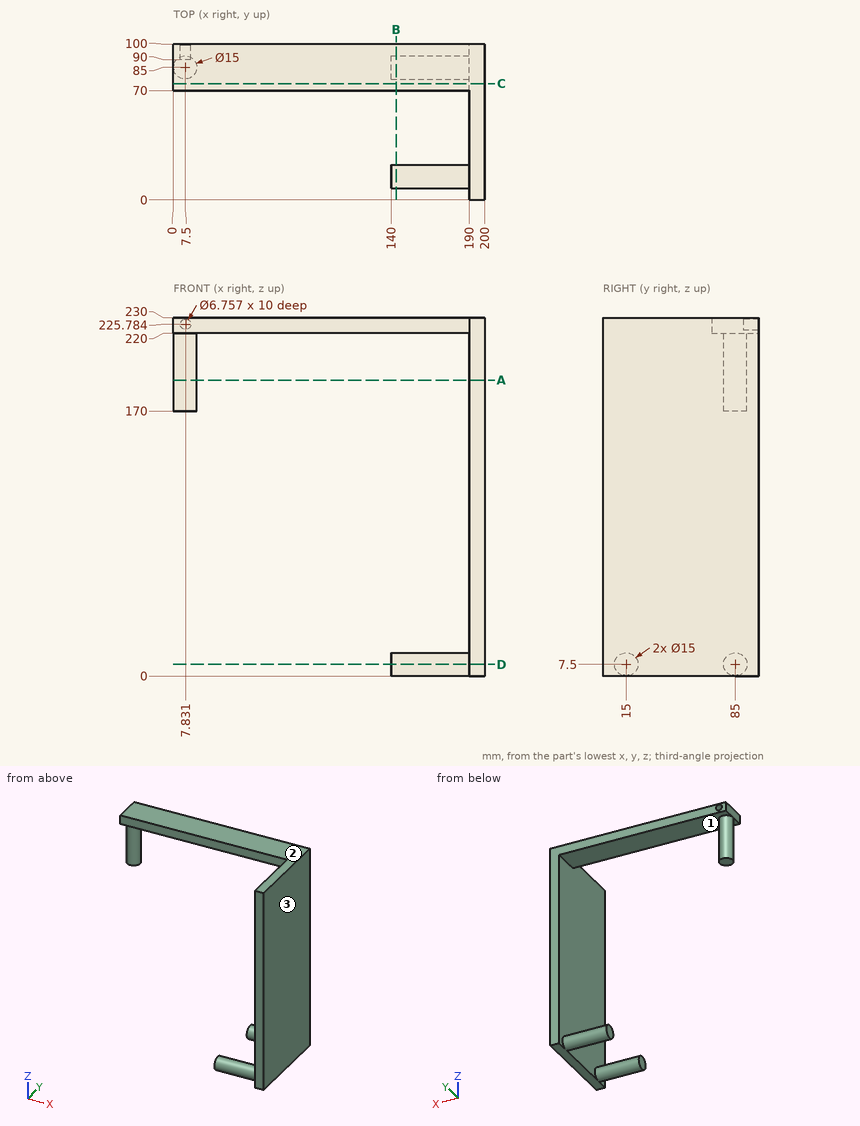
The drawing under review shows one solid part. Ordinate dimensions are in mm from its lowest x, y, z. Give positions to 0.01 mm unless a question says otherwise; leave off trailing zeros. Write each loop counter-clockwise with the first axis right and the second up, starting at its lowest first coordinate (ties: lowest second). Pieces come first, ordered by that corner, then holes. Notation, with made-up numbers: M 66.5,87 L 72.5,87 A10 ccw 72.5,92 Z; hole C 79,-6.5 d3. An arc over 180 degrees is marked long. Write each question's results on one line, items separated by ' | '. Start each with the question number.
1. We need section A-A (z = 190). Write out the cut boundary in (x, y), and give its area (3 significant figures).
2. We need section D-D (z = 7.5). Write out the cut boundary in (x, y).
3. Insertion check: pin 1 Ø7.5 at (y, z) = (84.5, 8.5) entering from -X; pin 2 Ø7.5 at (x, y) = (6, 88) entering from -Z; pin 3 Ø5.5 at (x, z) = (8, 227.5) entering from +Y; pin 4 Ø5 at (x, y) = (165, 26) entering from +Z. Each pin has a flat end and moves straight along its axis. Give the tip position at first contact, or say it passes through.
4. We need section B-B (x = 143). Write out the cut boundary in (y, z).
5. Mouldability with a two-part tool opening along X and no side actions: class the marked faces 1, 2 and 3 as released by +X, released by -X, zero draft, split by the parting line, or undercut.
6. For probe 1 along Z at (x, y) = (168, 84.5); probe 2 along X at (y, z) = (73, 114.5); probe 3 along Z at (x, y) = (14, 92), list the stretches that pass through material, from the lowest coordinate up. Write a range as [from, to].
7. We need section C-C (y = 74.5). Write out the cut boundary in (x, z).
Results found:
1) outline: C 7.5,85 d15; M 190,0 L 200,0 L 200,100 L 190,100 Z | area: 1,180 mm^2
2) outline: M 140,7.5 L 190,7.5 L 190,0 L 200,0 L 200,100 L 190,100 L 190,92.5 L 140,92.5 L 140,77.5 L 190,77.5 L 190,22.5 L 140,22.5 Z
3) pin 1: stops at x = 140 | pin 2: stops at z = 170 | pin 3: stops at y = 100 | pin 4: passes through
4) outline: C 15,7.5 d15; M 70,220 L 100,220 L 100,230 L 70,230 Z; C 85,7.5 d15
5) face 1: undercut | face 2: zero draft | face 3: released by +X
6) probe 1: z = [0.02, 14.98], [220, 230] | probe 2: x = [190, 200] | probe 3: z = [220, 230]
7) outline: M 0,220 L 190,220 L 190,0 L 200,0 L 200,230 L 0,230 Z
